Build history of the part. All positions in model axes, mm. A direction names the side the tool comes from. Round coordinates to 2 decimals unless told otherwise and drop trailing zeros. Order: outer loops, then holes, each group sorted by start corner. A loop starts at its lowest first (then second) coordinate and runs counter-clockwise, first axis right, second up. Notation, with made-up numbers: (66.25, -12) - (120.25, -12) arc R18 ccw to (120.25, 10) - close; hole circle Ø1 at (13.5, 15.25). An arc over 180 degrees is marked (long way). Write each question's results on one line, items separated by ' | '. Start each with the question number.
```python
from build123d import *

# Parameters (mm, degrees)
IZIM1_W                     = 36
IZIM1_H                     = 36
IZIM1_R                     = 8
Y_KSEKLIK_EKSTR_ZYON1_DEPTH = 50
IZIM2_W                     = 36
IZIM2_H                     = 5
KES_EKSTR_ZYON1_DEPTH       = 50
IZIM3_W                     = 36
IZIM3_H                     = 3
KES_EKSTR_ZYON2_DEPTH       = 50
KES_EKSTR_ZYON3_DEPTH       = 50
M4_BO_LUKLU_DELIK1_D        = 4.5
KES_EKSTR_ZYON5_START       = -50
KES_EKSTR_ZYON5_DEPTH       = 50


# Read off the part's stored shape, not the designer's step: Kes-Ekstrüzyon5
with BuildPart() as part:
    # Çizim1 → Yükseklik-Ekstrüzyon1 (new body)
    with BuildSketch(Plane.XY):
        Rectangle(IZIM1_W, IZIM1_H)
        Circle(IZIM1_R, mode=Mode.SUBTRACT)
    extrude(amount=Y_KSEKLIK_EKSTR_ZYON1_DEPTH)

    # Çizim2 → Kes-Ekstrüzyon1 (cut)
    with BuildSketch(Plane.XY.offset(50)):
        with Locations((0, 15.5)):
            Rectangle(IZIM2_W, IZIM2_H)
    extrude(amount=-KES_EKSTR_ZYON1_DEPTH, mode=Mode.SUBTRACT)

    # Çizim3 → Kes-Ekstrüzyon2 (cut)
    with BuildSketch(Plane.XY.offset(50)):
        with Locations((0, -16.5)):
            Rectangle(IZIM3_W, IZIM3_H)
    extrude(amount=-KES_EKSTR_ZYON2_DEPTH, mode=Mode.SUBTRACT)

    # Çizim4 → Kes-Ekstrüzyon3 (cut)
    with BuildSketch(Plane.XY.offset(50)):
        Polygon((-6.350852961, -11), (-9.526279442, -5.5), (-18, -5.5), (-18, -15), (18, -15), (18, -5.5), (9.526279442, -5.5), (6.350852961, -11), align=None)
    extrude(amount=-KES_EKSTR_ZYON3_DEPTH, mode=Mode.SUBTRACT)

    # M4 Boşluklu Delik1 (through all)
    with Locations(Plane(origin=(0, -5.5, 0), x_dir=(-1, 0, 0), z_dir=(0, -1, 0))):
        with Locations((-13.718329125, -40), (-13.718329125, -10), (12.810498521, -10), (12.810498521, -40)):
            Hole(M4_BO_LUKLU_DELIK1_D / 2)

    # Kes-Ekstrüzyon5 outline → Kes-Ekstrüzyon5 (cut)
    with BuildSketch(Plane.XY.offset(50).offset(KES_EKSTR_ZYON5_START)):
        with BuildLine():
            Line((7.066647013, 3.75), (18, 3.75))
            Line((18, 3.75), (18, 13))
            Line((18, 13), (-18, 13))
            Line((-18, 13), (-18, 3.75))
            Line((-18, 3.75), (-7.066647013, 3.75))
            ThreePointArc((-7.066647013, 3.75), (0, 8), (7.066647013, 3.75))
        make_face()
    extrude(amount=KES_EKSTR_ZYON5_DEPTH, mode=Mode.SUBTRACT)


solid = part.part
```
1. Cut at B-B (z = 10). List the corners of the cut face in (x, y), plus the area to 3 significant figures.
2. Flat gauge pins, fed straight in: pin 1 Ø9.5 at (x, z) = (12.5, 24.5) entering from -Y; pin 2 Ø7 at (x, z) = (-12.81, 40) entering from -Y; pin 3 Ø1 at (x, z) = (-3.5, 26.5) entering from +Y; pin 4 Ø4 at (x, z) = (13.72, 10) entering from -Y. Where does each tip first touch, or does it go through?
3. Cut at C-C (z = 46.5). List the corners of the cut face in (x, y).
4. Wall check: line 1 (X direction, y = 0, z = 38); line 2 (X direction, y = -3, z = 10); line 3 (X direction, y = 0, z = 15). Give the ranges that are in metal, low to high. Write a range as from..to.
5. 3-axis set-ups, long thin cutter, end or side, ignore diameter. For faces 1 (the face through (-13, 3.75, 25)), 2 (the face through (-14, -5.5, 25)), 3 (the face through (14, -5.5, 25)): which of +Z, -Z, +X, -X, +Y, -Y reach the whole face in a straight line?
6. Cut at D-D (y = -7.25). List the corners of the cut face in (x, z).
7. Cut at A-A (y = 0). List the corners of the cut face in (x, z), plus the area to 3 significant figures.
8. Mould opens along Z. For faces 4 (the face through (-18, -1, 25)), 5 (the face through (13.43, -0.81, 37.77)), 6 (the face through (-0.3, -8.4, 0)), 7 (the face through (12.06, -0.81, 8.48)) say: pulls with the +Z half, pulls with the -Z half, needs draft (parallel to the pull), parting line crosses it, or undercut.
A:
1) outline: (-18, -5.5) - (-15.06, -5.5) - (-15.06, 3.75) - (-18, 3.75) - close; (-10.56, -5.5) - (-9.53, -5.5) - (-6.35, -11) - (6.35, -11) - (9.53, -5.5) - (11.47, -5.5) - (11.47, 3.75) - (7.07, 3.75) arc R8 cw (long way) to (-7.07, 3.75) - (-10.56, 3.75) - close; (15.97, -5.5) - (18, -5.5) - (18, 3.75) - (15.97, 3.75) - close | area: 179 mm^2
2) pin 1: stops at y = -8.58 | pin 2: stops at y = -5.87 | pin 3: stops at y = -6.93 | pin 4: passes through
3) outline: (-18, -5.5) - (-9.53, -5.5) - (-6.35, -11) - (6.35, -11) - (9.53, -5.5) - (18, -5.5) - (18, 3.75) - (7.07, 3.75) arc R8 cw (long way) to (-7.07, 3.75) - (-18, 3.75) - close
4) line 1: x = -18..-13.84, -11.78..-8, 8..12.69, 14.75..18 | line 2: x = -18..-15.06, -10.56..-7.42, 7.42..11.47, 15.97..18 | line 3: x = -18..-8, 8..18
5) face 1: +Z, -Z, +X, -X, +Y | face 2: +Z, -Z, -X, -Y | face 3: +Z, -Z, +X, -Y
6) outline: (-8.52, 0) - (-3.38, 0) - (-3.38, 50) - (-8.52, 50) - close; (3.38, 0) - (8.52, 0) - (8.52, 50) - (3.38, 50) - close
7) outline: (-18, 0) - (-8, 0) - (-8, 50) - (-18, 50) - close; (8, 0) - (18, 0) - (18, 50) - (8, 50) - close; hole circle Ø4.5 at (-12.81, 10); hole circle Ø4.5 at (-12.81, 40); hole circle Ø4.5 at (13.72, 10); hole circle Ø4.5 at (13.72, 40) | area: 936 mm^2
8) face 4: needs draft | face 5: undercut | face 6: pulls with the -Z half | face 7: undercut
